CAD build for the part. Positions are in the model's coordinates, mm. Face numbers are marked on the shaded views. A direction names the side the tool comes from. Round coordinates to 2 decimals unless told otherwise and drop trailing zeros. Loops run counter-clockwise (first coordinate to the right, second up) from the corner with the lowest first, then second, coordinate; pieces in that order, holes last.
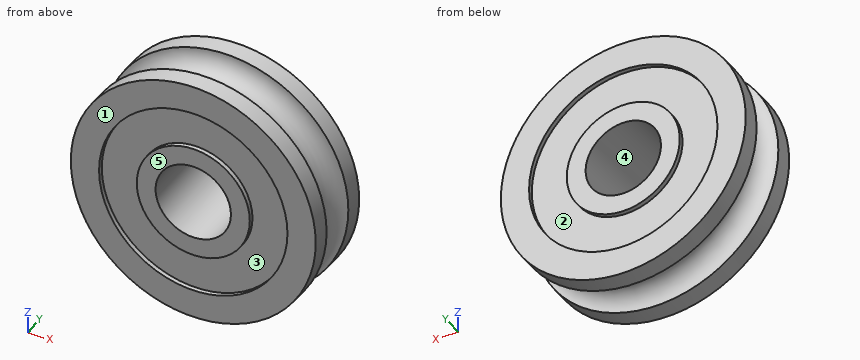
Autodesk Inventor part; units mm, degrees
ref_plane "YZ Plane" through (0, 0, 0) normal (1, 0, 0) x (0, 1, 0)
ref_plane "XZ Plane" through (0, 0, 0) normal (0, 1, 0) x (-1, 0, 0)
ref_plane "XY Plane" through (0, 0, 0) normal (0, 0, 1) x (1, 0, 0)
sketch "Sketch1" plane through (0, 0, 0) normal (0, 0, 1) x (1, 0, 0)
  line L0 (0, 0) -> (0, 5.0023) construction
  line L1 (2, 0) -> (6.5, 0)
  line L2 (6.5, 0) -> (6.5, 4)
  line L3 (6.5, 4) -> (2, 4)
  line L4 (2, 4) -> (2, 0)
  circle A0 centre (6.5, 2) radius 1
  line L5 (3, 4) -> (3, 3.75)
  line L6 (3, 3.75) -> (5, 3.75)
  line L7 (5, 3.75) -> (5, 4)
  line L8 (3, 0) -> (3, 0.25)
  line L9 (3, 0.25) -> (5, 0.25)
  line L10 (5, 0.25) -> (5, 0)
  point P0 (0, 2.5011)
  point P1 (6.5, 1)
  point P2 (6.5, 3)
  point P3 (3, 3.875)
  dimension "d0" = 2
  dimension "d1" = 2
  dimension "d2" = 6.5
  dimension "d3" = 4
  dimension "d5" = 0.25
  dimension "d6" = 1
  dimension "d7" = 2
revolve "Revolution1" add sketch "Sketch1" angle 360 about axis through (0, 0, 0) along (0, 1, 0) contours L4 L3 L5 L6 L7 L2 A0 L1 L10 L9 L8
properties part number "BearingU604" material "Steel, Alloy"
Item 1: 3-axis set-ups, long thin cutter, end or side, ignore diameter. For the marked faces 1, 2 and 3: which of +Z, -Z, +X, -X, +Y, -Y reach the whole face in a straight line?
Answers follow:
face 1: +Z, -Z, +X, -X, -Y
face 2: +Y
face 3: -Y
Item 2: Flat gauge pins, fed straight in: P1, Ø2, axis at y = 1, z = -4, coming from the -X side; P2, Ø1.5, axis at x = 1.5, y = 3, coming from the +Z side. Where does each tip first touch, or does it go through?
Answers follow:
P1: stops at x = -5.77
P2: stops at z = 6.46
Item 3: Probe line 1 (Z direction, x = 0, y = 3.85); line 2 (Y direction, x = -1.75, z = -4). List the from-to ranges inside material, lowest first.
Answers follow:
line 1: z = -6.5 to -5, -3 to -2, 2 to 3, 5 to 6.5
line 2: y = 0.25 to 3.75
Item 4: Cut at A-A, the plane z = 0. Give the cut face in (x, y).
Answers follow:
outline: (-6.5, 0) - (-5, 0) - (-5, 0.25) - (-3, 0.25) - (-3, 0) - (-2, 0) - (-2, 4) - (-3, 4) - (-3, 3.75) - (-5, 3.75) - (-5, 4) - (-6.5, 4) - (-6.5, 3) arc R1 cw to (-6.5, 1) - close; (2, 0) - (3, 0) - (3, 0.25) - (5, 0.25) - (5, 0) - (6.5, 0) - (6.5, 1) arc R1 cw to (6.5, 3) - (6.5, 4) - (5, 4) - (5, 3.75) - (3, 3.75) - (3, 4) - (2, 4) - close
Item 5: Cut at B-B, the plane x = 0. Give the cut face in (y, z).
Answers follow:
outline: (0, -6.5) - (1, -6.5) arc R1 cw to (3, -6.5) - (4, -6.5) - (4, -5) - (3.75, -5) - (3.75, -3) - (4, -3) - (4, -2) - (0, -2) - (0, -3) - (0.25, -3) - (0.25, -5) - (0, -5) - close; (0, 2) - (4, 2) - (4, 3) - (3.75, 3) - (3.75, 5) - (4, 5) - (4, 6.5) - (3, 6.5) arc R1 cw to (1, 6.5) - (0, 6.5) - (0, 5) - (0.25, 5) - (0.25, 3) - (0, 3) - close
Item 6: Cut at C-C, the plane y = 0.7. Give the cut face in (x, z).
Answers follow:
outline: circle Ø13 at (0, 0); hole circle Ø4 at (0, 0)
Item 7: Two-plate mould, pull along X, no slides. Class the marked faces 4 and 5: released by +X, released by -X, zero draft, split by the parting line, or undercut.
Answers follow:
face 4: undercut
face 5: zero draft
Item 8: Cut at D-D, the plane y = 2.8. Give the cut face in (x, z).
Answers follow:
outline: circle Ø11.8 at (0, 0); hole circle Ø4 at (0, 0)
